Autodesk Inventor part; units mm, degrees
ref_plane "YZ Plane" through (0, 0, 0) normal (1, 0, 0) x (0, 1, 0)
ref_plane "XZ Plane" through (0, 0, 0) normal (0, 1, 0) x (-1, 0, 0)
ref_plane "XY Plane" through (0, 0, 0) normal (0, 0, 1) x (1, 0, 0)
sketch "Sketch1" plane through (0, 0, 0) normal (0, 1, 0) x (-1, 0, 0)
  line L0 (0, 0) -> (63, 0)
  line L1 (63, 0) -> (63, -74)
  line L2 (63, -74) -> (0, -74)
  line L3 (0, -74) -> (0, 0)
  dimension "d0" = 63
  dimension "d1" = 74
extrude "Extrusion1" add sketch "Sketch1" along normal blind 25
sketch "Sketch2" plane through (0, 25, 0) normal (0, 1, 0) x (1, 0, 0)
  line L0 (-2, 2) -> (-61, 2)
  line L1 (-61, 2) -> (-61, 72)
  line L2 (-61, 72) -> (-2, 72)
  line L3 (-2, 72) -> (-2, 2)
  line L4 (-63, 74) -> (-63, 0)
  line L5 (-63, 0) -> (0, 0)
  line L6 (0, 0) -> (0, 74)
  dimension "d5" = 70
  dimension "d6" = 2
  dimension "d7" = 59
  dimension "d8" = 2
extrude "Extrusion2" cut sketch "Sketch2" against normal blind 23
sketch "Sketch3" plane through (0, 0, -74) normal (0, 0, -1) x (-1, 0, 0)
  line L0 (44, 17.5) -> (34, 17.5)
  line L1 (34, 17.5) -> (34, 10.5)
  line L2 (34, 10.5) -> (44, 10.5)
  line L3 (44, 10.5) -> (44, 17.5)
  line L4 (63, 0) -> (63, 25)
  line L5 (0, 25) -> (63, 25)
  point P0 (0, 0)
  dimension "d11" = 10
  dimension "d12" = 7
  dimension "d13" = 19
  dimension "d21" = 7.5
extrude "Extrusion3" cut sketch "Sketch3" against normal up to next
sketch "Sketch4" plane through (-63, 0, -74) normal (-1, 0, 0) x (0, 0, 1)
  circle A0 centre (66, 19) radius 3.25
  line L0 (74, 0) -> (74, 25)
  line L1 (0, 25) -> (74, 25)
  dimension "d16" = 6.5
  dimension "d17" = 8
  dimension "d18" = 6
extrude "Extrusion4" cut sketch "Sketch4" against normal up to next
sketch "Sketch5" plane through (-63, 0, 0) normal (0, 0, 1) x (1, 0, 0)
  circle A0 centre (23, 19) radius 4.25
  line L0 (29, 17.5) -> (29, 10.5)
  line L1 (0, 25) -> (63, 25)
  point P0 (63, 0)
  dimension "d22" = 8.5
  dimension "d23" = 6
  dimension "d24" = 6
extrude "Extrusion5" cut sketch "Sketch5" against normal up to next
sketch "Sketch6" plane through (0, 2, 0) normal (0, 1, 0) x (1, 0, 0)
  circle A0 centre (-4.5, 4.5) radius 2.5
  line L0 (0, 0) -> (0, 74)
  line L1 (-63, 0) -> (0, 0)
  circle A1 centre (-4.5, 69.5) radius 2.5
  line L2 (0, 74) -> (-63, 74)
  circle A2 centre (-58.5, 69.5) radius 2.5
  line L3 (-63, 74) -> (-63, 0)
  dimension "d27" = 5
  dimension "d28" = 4.5
  dimension "d29" = 4.5
  dimension "d30" = 5
  dimension "d31" = 4.5
  dimension "d32" = 5
  dimension "d33" = 4.5
extrude "Extrusion6" add sketch "Sketch6" along normal blind 21 contours A0 | A1 | A2
sketch "Sketch7" plane through (0, 23, 0) normal (0, 1, 0) x (1, 0, 0)
  arc A0 (-61, 69.5) -> (-58.5, 72) centre (-58.5, 69.5) ccw
  arc A1 (-4.5, 72) -> (-2, 69.5) centre (-4.5, 69.5) ccw
  arc A2 (-4.5, 72) -> (-2, 69.5) centre (-4.5, 69.5) ccw
  line L0 (-58.5, 72) -> (-4.5, 72)
  arc A3 (-61, 69.5) -> (-58.5, 72) centre (-58.5, 69.5) ccw
  line L1 (-61, 2) -> (-61, 69.5)
  line L2 (-4.5, 2) -> (-61, 2)
  arc A4 (-2, 4.5) -> (-4.5, 2) centre (-4.5, 4.5) ccw
  line L3 (-2, 69.5) -> (-2, 4.5)
  circle A5 centre (-4.5, 69.5) radius 1.5
  circle A6 centre (-58.5, 69.5) radius 1.5
  circle A7 centre (-4.5, 4.5) radius 1.5
  point P0 (0, 0)
  dimension "d36" = 3
  dimension "d37" = 3
  dimension "d38" = 3
extrude "Extrusion7" cut sketch "Sketch7" against normal blind 19 contours A5 | A6 | A7
sketch "Sketch8" plane through (0, 2, 0) normal (0, 1, 0) x (1, 0, 0)
  arc A0 (-4.5, 2) -> (-2, 4.5) centre (-4.5, 4.5) ccw
  line L0 (-4.5, 2) -> (-2, 2)
  line L1 (-2, 2) -> (-2, 4.5)
  line L2 (-2, 4.5) -> (-2, 4.1991)
  arc A1 (-4.5, 2) -> (-2, 4.5) centre (-4.5, 4.5) ccw
  arc A2 (-4.5, 72) -> (-2, 69.5) centre (-4.5, 69.5) ccw
  line L3 (-4.5, 72) -> (-2, 72)
  arc A3 (-2, 69.5) -> (-4.5, 72) centre (-4.5, 69.5) ccw
  line L4 (-2, 72) -> (-2, 69.5)
  arc A4 (-2, 69.5) -> (-4.5, 72) centre (-4.5, 69.5) ccw
  arc A5 (-58.5, 72) -> (-61, 69.5) centre (-58.5, 69.5) ccw
  arc A6 (-58.5, 72) -> (-61, 69.5) centre (-58.5, 69.5) ccw
  line L5 (-61, 69.5) -> (-61, 72)
  line L6 (-61, 72) -> (-58.5, 72)
  point P0 (0, 0)
extrude "Extrusion8" add sketch "Sketch8" along normal blind 21 contours A0 L1 L0 | L3 L4 A3 | A5 L5 L6
sketch "Sketch9" plane through (0, 25, 0) normal (0, 1, 0) x (1, 0, 0)
  point P0 (0, 0)
properties part number "bottom"
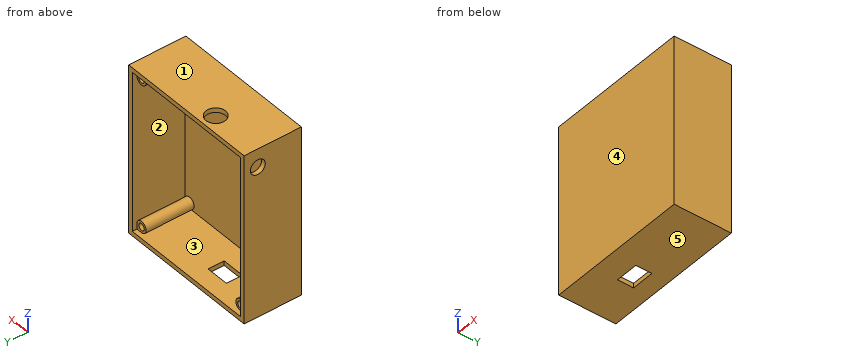
Work out the finished part from the listing and answer in its coordinate system (mm). Face numbers are marked on the shaded views. A direction names the side the tool comes from. Give positions to 0.01 mm unless a question says otherwise; leave off trailing zeros. Order: outer loops, then holes, each group sorted by start corner. A loop starts at its lowest first (then second) coordinate and runs counter-clockwise, first axis right, second up. Notation, with made-up numbers: M -24,-29.5 L 10,-29.5 A25 cw 10,-6.5 Z; hole C 12.25,-20 d7. An arc over 180 degrees is marked long. Return JSON: item names as keys, results as strings.
Q1. Find section C-C, the plane z = -8. Write down the section's boundary in (x, y), and give its area (3 significant figures).
Answer below:
{"outline": "M -63,0 L 0,0 L 0,25 L -2,25 L -2,2 L -61,2 L -61,15.75 L -63,15.75 Z; M -63,22.25 L -61,22.25 L -61,25 L -63,25 Z", "area": "205 mm^2"}
Q2. Find the intervals of material crossed by line 1 along Z through (x, y) = (-51, 12); line 2 along X through (y, z) = (20, -64); line 3 along Y through (x, z) = (-62, -8), in increasing order. Write a range as [from, to].
Answer below:
{"line 1": "z = [-74, -72], [-2, 0]", "line 2": "x = [-63, -61], [-2, 0]", "line 3": "y = [0, 15.75], [22.25, 25]"}
Q3. Find section D-D, the plane z = -48.5. Write down the section's boundary in (x, y).
Answer below:
{"outline": "M -63,0 L 0,0 L 0,25 L -2,25 L -2,2 L -61,2 L -61,25 L -63,25 Z"}
Q4. The mould has two halves that part along Z. Classify the marked faces 3, 4 and 5: pulls with the +Z half, pulls with the -Z half, needs draft (parallel to the pull), parting line crosses it, or undercut.
Answer below:
{"face 3": "undercut", "face 4": "needs draft", "face 5": "pulls with the -Z half"}
Q5. Find section B-B, the plane x = -40. Write down the section's boundary in (y, z), and give its area (3 significant figures).
Answer below:
{"outline": "M 0,-74 L 10.5,-74 L 10.5,-72 L 2,-72 L 2,-2 L 14.75,-2 L 14.75,0 L 0,0 Z; M 17.5,-74 L 25,-74 L 25,-72 L 17.5,-72 Z; M 23.25,-2 L 25,-2 L 25,0 L 23.25,0 Z", "area": "209 mm^2"}
Q6. Which of the six approach directions +Z, -Z, +X, -X, +Y, -Y give full straight-line access (tool end or side, diameter ignored) to the marked faces 1 and 2?
Answer below:
{"face 1": "+Z, +X, -X, +Y, -Y", "face 2": "+Y"}
Q7. Each of these flat-tipped pins is pushed along its axis until it touches: pin 1 (1.5 mm diameter, centred on x = -58.5, z = -70, fed in from +Y); pin 2 (5 mm diameter, centred on x = -11, z = -51.5, fed in from +Y); pin 3 (3.5 mm diameter, centred on x = -4, z = -4.5, fed in from +Y). Where does it stop, or does it pass through?
Answer below:
{"pin 1": "stops at y = 4", "pin 2": "stops at y = 2", "pin 3": "stops at y = 23"}
Q8. Find section A-A, the plane y = 19. Write down the section's boundary in (x, z).
Answer below:
{"outline": "M -63,-74 L 0,-74 L 0,0 L -35.75,0 L -35.75,-2 L -4.5,-2 A2.5 ccw long -2,-4.5 L -2,-69.5 A2.5 ccw long -4.5,-72 L -58.5,-72 A2.5 ccw long -61,-69.5 L -61,-11.25 L -63,-11.25 Z; M -63,-4.75 L -61,-4.75 L -61,-2 L -44.25,-2 L -44.25,0 L -63,0 Z; hole C -58.5,-69.5 d3; hole C -4.5,-69.5 d3; hole C -4.5,-4.5 d3"}
